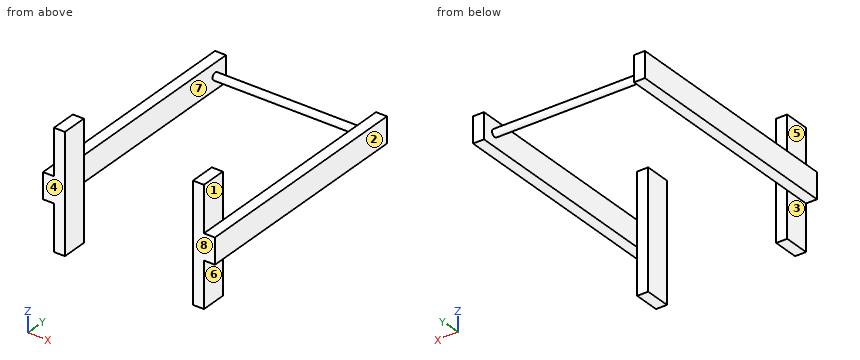
Autodesk Inventor part; units mm, degrees
ref_plane "YZ Plane" through (0, 0, 0) normal (1, 0, 0) x (0, 1, 0)
ref_plane "XZ Plane" through (0, 0, 0) normal (0, 1, 0) x (-1, 0, 0)
ref_plane "XY Plane" through (0, 0, 0) normal (0, 0, 1) x (1, 0, 0)
sketch "Sketch1" plane through (0, 0, 0) normal (0, 1, 0) x (-1, 0, 0)
  line L0 (0, -284.48) -> (0, 284.48)
  line L1 (-364.49, 0) -> (364.49, 0)
  line L2 (260.35, 203.2) -> (222.25, 203.2)
  line L3 (222.25, 203.2) -> (222.25, -203.2)
  line L4 (222.25, -203.2) -> (260.35, -203.2)
  line L5 (260.35, -203.2) -> (260.35, 203.2)
  line L6 (260.35, 203.2) -> (222.25, -203.2) construction
  line L7 (222.25, 203.2) -> (260.35, -203.2) construction
  line L8 (-260.35, 203.2) -> (-222.25, 203.2)
  line L9 (-222.25, 203.2) -> (-222.25, -203.2)
  line L10 (-222.25, -203.2) -> (-260.35, -203.2)
  line L11 (-260.35, -203.2) -> (-260.35, 203.2)
  line L12 (-260.35, 203.2) -> (-222.25, -203.2) construction
  line L13 (-222.25, 203.2) -> (-260.35, -203.2) construction
  point P0 (0, 0)
  point P1 (241.3, 0)
  point P2 (-241.3, 0)
  dimension "d0" = 38.1
  dimension "d1" = 406.4
  dimension "d3" = 260.35
extrude "Extrusion1" add sketch "Sketch1" along normal blind 88.9
sketch "Sketch2" plane through (0, 0, 0) normal (0, -1, 0) x (1, 0, 0)
  line L0 (-260.35, 203.2) -> (-222.25, 203.2)
  line L1 (-260.35, -203.2) -> (-260.35, 203.2)
  line L2 (-222.25, -203.2) -> (-260.35, -203.2)
  line L3 (-222.25, 203.2) -> (-222.25, -203.2)
  line L4 (260.35, 203.2) -> (222.25, 203.2)
  line L5 (222.25, 203.2) -> (222.25, -203.2)
  line L6 (222.25, -203.2) -> (260.35, -203.2)
  line L7 (260.35, -203.2) -> (260.35, 203.2)
  line L8 (-417.83, 0) -> (417.83, 0)
  line L9 (-298.45, -44.45) -> (-260.35, -44.45)
  line L10 (-260.35, -44.45) -> (-260.35, 44.45)
  line L11 (-260.35, 44.45) -> (-298.45, 44.45)
  line L12 (-298.45, 44.45) -> (-298.45, -44.45)
  line L13 (-298.45, -44.45) -> (-260.35, 44.45) construction
  line L14 (-260.35, -44.45) -> (-298.45, 44.45) construction
  line L15 (0, 284.48) -> (0, -284.48)
  line L16 (298.45, -44.45) -> (260.35, -44.45)
  line L17 (260.35, -44.45) -> (260.35, 44.45)
  line L18 (260.35, 44.45) -> (298.45, 44.45)
  line L19 (298.45, 44.45) -> (298.45, -44.45)
  line L20 (298.45, -44.45) -> (260.35, 44.45) construction
  line L21 (260.35, -44.45) -> (298.45, 44.45) construction
  point P0 (0, 0)
  point P1 (-279.4, 0)
  point P2 (279.4, 0)
  dimension "d6" = 38.1
  dimension "d7" = 88.9
extrude "Extrusion2" add sketch "Sketch2" against normal blind 812.8 contours L1 L8 L12 L11 | L1 L9 L12 L8 | L8 L19 L16 L7 | L7 L18 L19 L8
sketch "Sketch3" plane through (298.45, 0, 44.45) normal (1, 0, 0) x (0, 0, -1)
  line L0 (88.9, 0) -> (0, 0)
  line L1 (88.9, 0) -> (88.9, 812.8)
  line L2 (0, 812.8) -> (88.9, 812.8)
  line L3 (0, 0) -> (0, 812.8)
  line L4 (44.45, -162.56) -> (44.45, 975.36)
  circle A0 centre (44.45, 762) radius 12.7
  point P0 (44.45, 0)
  dimension "d10" = 25.4
  dimension "d11" = 762
extrude "Extrusion3" add sketch "Sketch3" against normal up to surface (596.9 mm away) contours A0 L4 | L4 A0
properties part number "Perch"
The listing builds one solid part. Answer for the finished solid, in the listing's coordinates (mm). Face numbers are marked on the shaded views. A direction names the side the tool comes from. Round coordinates to 2 decimals unless told otherwise and drop trailing zeros. Write each loop counter-clockwise with the first axis right and the second up, starting at its lowest first coordinate (ties: lowest second). Pieces come first, ordered by that corner, then holes. Notation, with made-up numbers: (75.25, -34.5) -> (89.25, -34.5) arc R5 cw to (89.25, -29.5) -> close; hole circle Ø1 at (15, 36.5). An arc over 180 degrees is marked (long way). Use CSV: the item, a comma, the result in double quotes. Start each with the question number.
(1) Each of these flat-tipped pins is pushed along its axis until it touches: pin 1 (19 mm diameter, centred on x = 287, y = 555, fed in from +Z); pin 2 (19 mm diameter, centred on x = 234.5, z = -100.5, fed in from +Y). Where does it stop, or does it pass through?
(2) Section C-C on x = -241.5 is taken. Give the vertices of the cut face in (y, z), then the cut area to 3 significant figures.
(3) Consider L1, parallel to X at y = 34.5, z = 39; L2, parallel to X at y = 136, z = 28.5; L3, parallel to Y at x = 251, z = 55. Determine where each line is inside the solid, lowest interval first. Write a range as from..to.
(4) Section A-A on z = -134 is taken. Give the vertices of the cut face in (x, y), then the cut area to 3 significant figures.
(5) Section D-D on z = 0 is taken. Give the vertices of the cut face in (x, y), then the cut area to 3 significant figures.
(6) Which of the six approach directions +Z, -Z, +X, -X, +Y, -Y give full straight-line access (tool end or side, diameter ignored) to the marked faces 1, 2, 3, 4 and 5?
(7) Section B-B on y = 669 is taken. Give the vertices of the cut face in (x, z), then the cut area to 3 significant figures.
(8) The mould has two halves that part along X. Classify the marked faces 6, 7 and 8: released by +X, released by -X, zero draft, split by the parting line, or undercut.
A:
1,pin 1,"stops at z = 44.45"
1,pin 2,"stops at y = 88.9"
2,outline,"(0, -203.2) -> (88.9, -203.2) -> (88.9, 203.2) -> (0, 203.2) -> close; circle Ø25.4 at (762, 0)"
2,area,"36,600 mm²"
3,L1,"x = -298.45..-222.25, 222.25..298.45"
3,L2,"x = -298.45..-260.35, 260.35..298.45"
3,L3,"y = 0..88.9"
4,outline,"(-260.35, 0) -> (-222.25, 0) -> (-222.25, 88.9) -> (-260.35, 88.9) -> close; (222.25, 0) -> (260.35, 0) -> (260.35, 88.9) -> (222.25, 88.9) -> close"
4,area,"6,770 mm²"
5,outline,"(-298.45, 0) -> (-222.25, 0) -> (-222.25, 88.9) -> (-260.35, 88.9) -> (-260.35, 749.3) -> (260.35, 749.3) -> (260.35, 88.9) -> (222.25, 88.9) -> (222.25, 0) -> (298.45, 0) -> (298.45, 812.8) -> (260.35, 812.8) -> (260.35, 774.7) -> (-260.35, 774.7) -> (-260.35, 812.8) -> (-298.45, 812.8) -> close"
5,area,"81,900 mm²"
6,face 1,"+Z, +X, +Y, -Y"
6,face 2,"+Z, -Z, +X, +Y, -Y"
6,face 3,"-Z, -X, +Y, -Y"
6,face 4,"+Z, -Z, +X, -X, -Y"
6,face 5,"+Z, -X, +Y, -Y"
7,outline,"(-298.45, -44.45) -> (-260.35, -44.45) -> (-260.35, 44.45) -> (-298.45, 44.45) -> close; (260.35, -44.45) -> (298.45, -44.45) -> (298.45, 44.45) -> (260.35, 44.45) -> close"
7,area,"6,770 mm²"
8,face 6,"released by +X"
8,face 7,"undercut"
8,face 8,"zero draft"
